```python
from build123d import *

# Parameters (mm, degrees)
ESQUISSE1_W                                       = 50
ESQUISSE1_H                                       = 50
ESQUISSE1_R                                       = 1
BOSS_EXTRU_1_DEPTH                                = 5
FRAISAGE_POUR_VIS_T_TE_FRAIS_E_M31_D              = 3.4
FRAISAGE_POUR_VIS_T_TE_FRAIS_E_M31_CSINK_D        = 6.3
FRAISAGE_POUR_VIS_T_TE_FRAIS_E_M31_CSINK_ANGLE    = 90
FRAISAGE_POUR_VIS_T_TE_FRAIS_E_M31_ON_D           = 3.4
FRAISAGE_POUR_VIS_T_TE_FRAIS_E_M31_ON_CSINK_D     = 6.3
FRAISAGE_POUR_VIS_T_TE_FRAIS_E_M31_ON_CSINK_ANGLE = 90


with BuildPart() as part:
    # Esquisse1 → Boss.-Extru.1 (new body)
    with BuildSketch(Plane.XY):
        with Locations((-13.443105546, 23.082518784)):
            Rectangle(ESQUISSE1_W, ESQUISSE1_H)
        with Locations((-35.443105546, 45.082518784)):
            Circle(ESQUISSE1_R, mode=Mode.SUBTRACT)
        with Locations((8.556894454, 45.082518784)):
            Circle(ESQUISSE1_R, mode=Mode.SUBTRACT)
        with Locations((8.556894454, 1.082518784)):
            Circle(ESQUISSE1_R, mode=Mode.SUBTRACT)
        with Locations((-35.443105546, 1.082518784)):
            Circle(ESQUISSE1_R, mode=Mode.SUBTRACT)
    extrude(amount=BOSS_EXTRU_1_DEPTH)

    # Fraisage pour vis à tête fraisée M31 (through all)
    with Locations(Plane(origin=(-13.443105546, 38.082518784, 5), x_dir=(1, 0, 0), z_dir=(0, 0, 1))):
        with Locations((0, 0), (15, 0)):
            CounterSinkHole(FRAISAGE_POUR_VIS_T_TE_FRAIS_E_M31_D / 2, FRAISAGE_POUR_VIS_T_TE_FRAIS_E_M31_CSINK_D / 2, counter_sink_angle=FRAISAGE_POUR_VIS_T_TE_FRAIS_E_M31_CSINK_ANGLE)

    # Fraisage pour vis à tête fraisée M31 on (through all)
    with Locations(Plane(origin=(-69.932791176, 61.393115675, 0), x_dir=(1, 0, 0), z_dir=(0, 0, 1))):
        with Locations((0, 0)):
            CounterSinkHole(FRAISAGE_POUR_VIS_T_TE_FRAIS_E_M31_ON_D / 2, FRAISAGE_POUR_VIS_T_TE_FRAIS_E_M31_ON_CSINK_D / 2, counter_sink_angle=FRAISAGE_POUR_VIS_T_TE_FRAIS_E_M31_ON_CSINK_ANGLE)


solid = part.part
```
Check sheet for the modelled part. Datum: model origin and axes. Units: mm. Coordinates: 2 decimals unless noted, no trailing zeros. Write each question's results on one line, items separated by ' | '. Start each with the question number.
1) Depth check by flat-ended pin: pin 1 (3 mm diameter, centred on x = 1.56, y = 38.08, fed in from -Z); pin 2 (5 mm diameter, centred on x = -23.5, y = 35, fed in from -Z). Enter the tip coordinate at first touch or a pass-through.
2) Draft check along X on faces 1 (the face through (11.557, 23, 2)), 2 (the face through (-12.19, 39.23, 1.75)), 3 (the face through (-14, 23, 0)). Enter one of: pulls with the +X half, pulls with the -X half, needs draft (parallel to the pull), parting line crosses it, or undercut.
3) Section check A-A (y = 39). Count the separate pieces of the cut face and the enclosed holes in it, and give its area (3 significant figures).
4) Material ranges on line 1 along Y through (x, z) = (2.5, 3.9); line 2 along Y through (x, z) = (8, 0.75); line 3 along Y through (x, z) = (-15, 2.8), recorded low to high.
Checked values:
1) pin 1: through | pin 2: z = 0
2) face 1: pulls with the +X half | face 2: undercut | face 3: needs draft
3) separate pieces: 3 | enclosed holes: 0 | area: 217 mm²
4) line 1: -1.92 to 36.26, 39.9 to 48.08 | line 2: -1.92 to 0.25, 1.91 to 44.25, 45.91 to 48.08 | line 3: -1.92 to 37.4, 38.77 to 48.08
